Source: CAD feature listing. Evaluate the final solid. Frame: model axes, mm. Face numbers are marked on the shaded views. A direction names the side the tool comes from. Round coordinates to 2 decimals unless told otherwise and drop trailing zeros. Order: outer loops, then holes, each group sorted by start corner. A loop starts at its lowest first (then second) coordinate and runs counter-clockwise, first axis right, second up. Notation, with made-up numbers: (-1.75, -23) -> (37.25, -23) arc R21 ccw to (37.25, 0) -> close; hole circle Ø11 at (-20, 48). An arc over 180 degrees is marked (long way). Use a Markdown table: item, result. Add a question column.
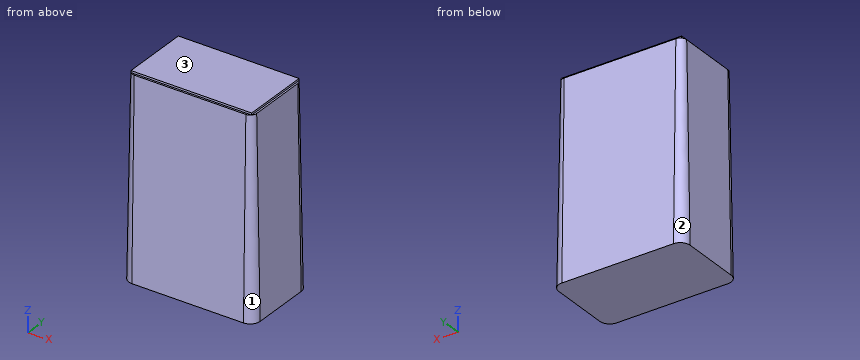
```python
from build123d import *

# Parameters (mm, degrees)
EXTRUDE_1_DEPTH  = 300
EXTRUDE_1_TAPER  = 1
SHELL_1_T        = -4
EXTRUDE_2_DEPTH  = 60
SKETCH_5_W       = 90.762871209
SKETCH_5_H       = 50.762871209
EXTRUDE_3_DEPTH  = 3
EXTRUDE_4_DEPTH  = 3
SKETCH_8_W       = 183.80764657
SKETCH_8_H       = 103.80764657
EXTRUDE_11_DEPTH = 3


with BuildPart() as part:
    # 草图1 → 凸台-拉伸1 (new body)
    with BuildSketch(Plane.XY):
        with BuildLine():
            ThreePointArc((-85, 60), (-95.606601718, 55.606601718), (-100, 45))
            Line((-100, 45), (-100, -45))
            ThreePointArc((-100, -45), (-95.606601718, -55.606601718), (-85, -60))
            Line((-85, -60), (85, -60))
            ThreePointArc((85, -60), (95.606601718, -55.606601718), (100, -45))
            Line((100, -45), (100, 45))
            ThreePointArc((100, 45), (95.606601718, 55.606601718), (85, 60))
            Line((85, 60), (-85, 60))
        make_face()
    extrude(amount=EXTRUDE_1_DEPTH, taper=EXTRUDE_1_TAPER)

    # 抽壳1
    shell_1_openings = [part.faces().sort_by_distance(p)[0] for p in [
        (0, 0, 300),
    ]]
    offset(amount=SHELL_1_T, openings=shell_1_openings, kind=Kind.INTERSECTION)

    # 草图4 → 凸台-拉伸2 (add)
    with BuildSketch(Plane.XY.offset(4)):
        Polygon((0, 0.466595392), (0, 0), (0, -0.395363651), (2.934231711, -0.395363651), (2.934231711, 0), (2.934231711, 50.762871209), (0, 50.762871209), align=None)
    extrude_2 = extrude(amount=EXTRUDE_2_DEPTH)

    # 草图5 → 凸台-拉伸3 (add)
    with BuildSketch(Plane(origin=(6.01372394, 0, 64), x_dir=(1, 0, 0), z_dir=(0, 0, 1))):
        with Locations((45.381435605, 25.381435605)):
            Rectangle(SKETCH_5_W, SKETCH_5_H)
    extrude_3 = extrude(amount=EXTRUDE_3_DEPTH)

    # 草图6 → 凸台-拉伸4 (add)
    with BuildSketch(Plane.XY.offset(64)):
        Polygon((0, 25.183753779), (6.01372394, 28.76636796), (6.01372394, 21.601139598), align=None)
    extrude(amount=EXTRUDE_4_DEPTH)

    # 镜向1: 凸台-拉伸2, 凸台-拉伸3 across plane
    add(extrude_2.mirror(Plane(origin=(0, -0.395363651, 64), x_dir=(0, 0, 1), z_dir=(0, -1, 0))))
    add(extrude_3.mirror(Plane(origin=(0, -0.395363651, 64), x_dir=(0, 0, 1), z_dir=(0, -1, 0))))

    # 草图8 → 凸台-拉伸11 (add)
    with BuildSketch(Plane.XY.offset(300)):
        Rectangle(SKETCH_8_W, SKETCH_8_H)
    extrude(amount=EXTRUDE_11_DEPTH)


solid = part.part
```
1) Reachability of the marked faces 1, 2 and 3 from +Z, -Z, +X, -X, +Y, -Y: full face, straight path, thin tool, end or side. Return the list, or none.
2) First-contact query: pin 1 Ø2.5 at (x, z) = (50, 65.5) entering from -Y; pin 2 Ø4 at (y, z) = (9.5, 113.5) entering from +X; pin 3 Ø15 at (x, y) = (30, 20.5) entering from -Z; pin 4 Ø2 at (x, z) = (15, 250) entering from +Y. Flat tips, straight axial feed; report the tip coordinate or a pass-through.
3) Section C-C on y = 12.5. Output: boundary loops of the cut face in (x, z), then the cut area to 3 significant figures.
4) Line query: probe 1 along Z at (x, y) = (15, -33.5); probe 2 along Y at (x, z) = (-0.5, 233.5); probe 3 along X at (y, z) = (4, 237). Output: solid intervals per line, ascending. Write a range as from..to.
5) Section B-B on z = 32.5. Output: boundary loops of the cut face in (x, y).
6) Section D-D on x = -40.5. Output: boundary loops of the cut face in (y, z), then the cut area to 3 significant figures.
7) Section A-A on x = 18. Output: boundary loops of the cut face in (y, z), then the cut area to 3 significant figures.
Conclusion:
| question | item | result |
|---|---|---|
| 1 | face 1 | +Z, +X, -Y |
| 1 | face 2 | +Z, -X, +Y |
| 1 | face 3 | +Z, +X, -X, +Y, -Y |
| 2 | pin 1 | stops at y = -58.88 |
| 2 | pin 2 | stops at x = 98.05 |
| 2 | pin 3 | stops at z = 0 |
| 2 | pin 4 | stops at y = 55.65 |
| 3 | outline | (-100, 0) -> (100, 0) -> (94.76, 300) -> (91.9, 300) -> (91.9, 303) -> (-91.9, 303) -> (-91.9, 300) -> (-94.76, 300) -> close; hole (-95.93, 4) -> (0, 4) -> (0, 64) -> (2.93, 64) -> (2.93, 4) -> (95.93, 4) -> (94.88, 64) -> (6.01, 64) -> (6.01, 67) -> (94.83, 67) -> (90.76, 300) -> (-90.76, 300) -> close |
| 3 | area | 4,160 mm^2 |
| 4 | probe 1 | z = 0..4, 64..67, 300..303 |
| 4 | probe 2 | y = -55.92..-51.92, 51.92..55.92 |
| 4 | probe 3 | x = -95.86..-91.86, 91.86..95.86 |
| 5 | outline | (-99.43, -45) arc R14.43 ccw to (-85, -59.43) -> (85, -59.43) arc R14.43 ccw to (99.43, -45) -> (99.43, 45) arc R14.43 ccw to (85, 59.43) -> (-85, 59.43) arc R14.43 ccw to (-99.43, 45) -> close; (0, -51.55) -> (2.93, -51.55) -> (2.93, 50.76) -> (0, 50.76) -> close; hole (-95.43, -45) arc R10.43 ccw to (-85, -55.43) -> (85, -55.43) arc R10.43 ccw to (95.43, -45) -> (95.43, 45) arc R10.43 ccw to (85, 55.43) -> (-85, 55.43) arc R10.43 ccw to (-95.43, 45) -> close |
| 6 | outline | (-60, 0) -> (60, 0) -> (54.76, 300) -> (51.9, 300) -> (51.9, 303) -> (-51.9, 303) -> (-51.9, 300) -> (-54.76, 300) -> close; hole (-55.93, 4) -> (55.93, 4) -> (50.76, 300) -> (-50.76, 300) -> close |
| 6 | area | 3,160 mm^2 |
| 7 | outline | (-60, 0) -> (60, 0) -> (54.76, 300) -> (51.9, 300) -> (51.9, 303) -> (-51.9, 303) -> (-51.9, 300) -> (-54.76, 300) -> close; (-51.55, 64) -> (-0.79, 64) -> (-0.79, 67) -> (-51.55, 67) -> close; (0, 64) -> (50.76, 64) -> (50.76, 67) -> (0, 67) -> close; hole (-55.93, 4) -> (55.93, 4) -> (50.76, 300) -> (-50.76, 300) -> close |
| 7 | area | 3,460 mm^2 |
